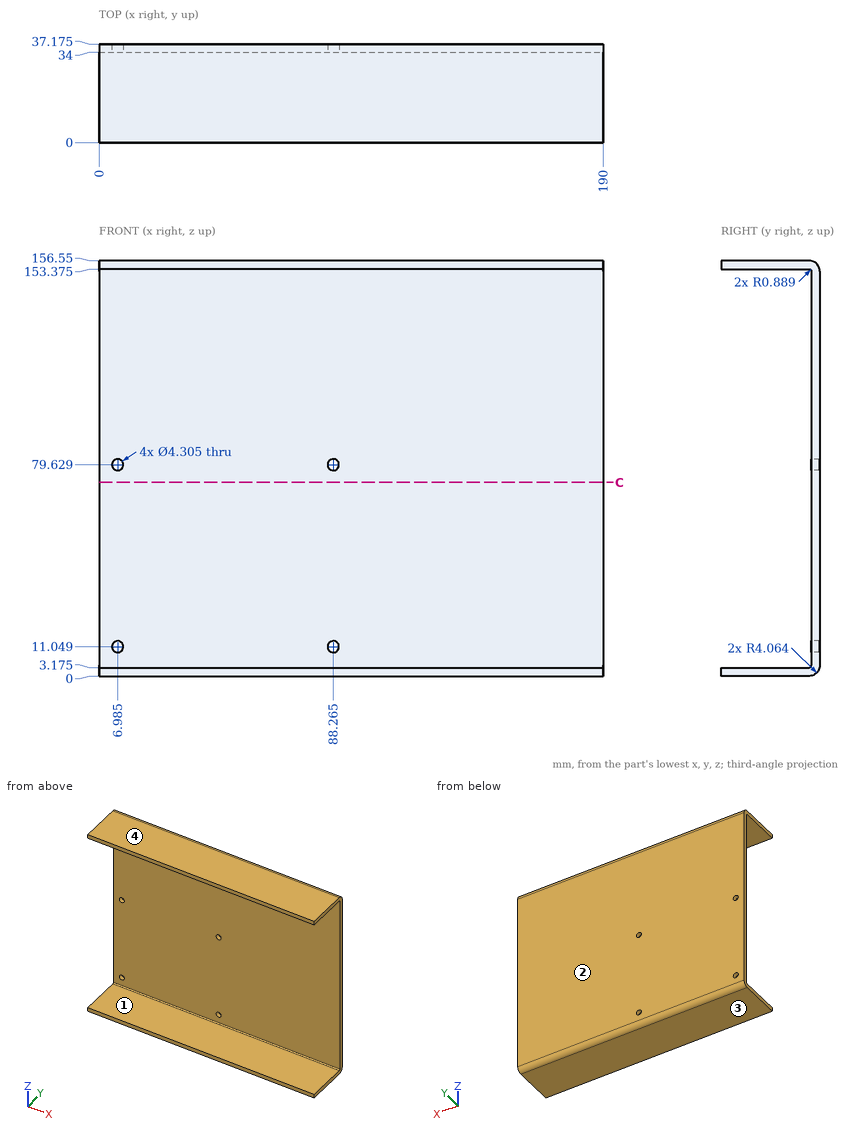
Design review of the part shown in the three views and the two pictorial views. Dimensions are in mm from the part's minimum x, y and z. Give positions to 0.01 mm unless a question says otherwise; leave off trailing zeros. Write each loop counter-clockwise with the first axis right and the second up, starting at its lowest first coordinate (ties: lowest second). Pieces come first, ordered by that corner, then holes.
(1) Add section C-C (z = 73). Give the boundary of the cut face in (x, y) (1 decimal), and give its area (3 significant figures).
Checked values:
outline: (0, 34) - (190, 34) - (190, 37.2) - (0, 37.2) - close
area: 603 mm2
(2) Clearance check with flat-ended pins moving along their axes: pin 1 Ø4 at (x, z) = (43, 121.5) entering from -Y; pin 2 Ø4 at (x, z) = (6.985, 11.049) entering from +Y. State where each tip first meets the part, or that it passes through.
Checked values:
pin 1: stops at y = 34
pin 2: passes through
(3) Wall thickness on line 1 along Y through (x, z) = (21, 139.5) (1 decimal); line 2 along Z through (x, y) = (147.5, 35) (1 decimal): over which ranges is each line inside the solid? List them lowest first.
Checked values:
line 1: y = 34 to 37.2
line 2: z = 0.5 to 156.1
(4) Mouldability with a two-part tool opening along Z and no side actions: class the marked faces 1, 2, 3 and 4 as +Z half, -Z half, draft (parallel to the pull), parting line (faces both ways), or undercut.
Checked values:
face 1: undercut
face 2: draft
face 3: -Z half
face 4: +Z half
